Input: part model. Units: mm. Frame: model coordinates. A direction names the side the tool comes from. Give positions to 0.01 mm unless a question says otherwise; leave off trailing zeros. Order: outer loops, then holes, each group sorted by start corner. A loop starts at its lowest first (then second) coordinate and runs counter-clockwise, first axis right, second up. Notation, with made-up numbers: (-9.75, 55.25) - (3.25, 55.25) arc R23 cw to (3.25, 92.25) - close; hole circle Ø3 at (51.25, 19.25). An arc over 180 degrees is marked (long way). Answer in a Markdown table with one row per item. Add a question column.
1. Section query D-D on z = 7.5. Return loops of the section in (x, y).
2. Access query for faces 5 (the face through (0, -4, -10)), 6 (the face through (-0.13, -7.99, 8.49)), 7 (the face through (4.25, -4, 0)), 8 (the face through (-4.25, -4, 0)). Directions: +Z, -Z, +X, -X, +Y, -Y. A direction counts if a zero-diameter tool reaches every point of the face in a straight line with its end or side. Return the directions, or none.
3. Contact query for flat-ended pins moving along their axis: pin 1 (1.7 mm diameter, centred on y = -4, z = 2.5, fed in from +X); pin 2 (12 mm diameter, centred on x = 3.5, z = -5.5, fed in from -Y); pin 3 (12 mm diameter, centred on x = 4.5, z = -0.5, fed in from -Y); pin 4 (1 mm diameter, centred on x = -1.5, y = -6.5, fed in from -Z). Output: stop coordinate, or through.
4. Ray query, line 1 (Y direction, x = 9.5, z = 0); line 2 (Z direction, x = -1, y = -6); line 3 (X direction, y = -6, z = -8.25). Return the intervals inside material, ascending. Write a range as [from, to].
5. Section query B-B on x = 0. Return loops of the section in (y, z).
6. Mould query, pull axis Z, two halves, no side actions, for faces 1 (the face through (0, -4, 10)), 2 (the face through (6.586, -0.592, 10.329)), 3 (the face through (-0.13, -7.99, -6.51)), 4 (the face through (0, 0, 0)). Classes: released by +Z, released by -Z, zero draft, split by the parting line, or undercut.
7. Section query C-C on y = -3.25. Return loops of the section in (x, z).
8. Section query A-A on z = 0. Return loops of the section in (x, y).
```python
from build123d import *

# Parameters (mm, degrees)
F0_R     = 12.25
F0_W     = 8.5
F0_H     = 20
F1_DEPTH = 1.2
F0_R_2   = 1
F2_DEPTH = 7
F3_DEPTH = 9


with BuildPart() as f1:
    # F0 (on Front) → F1 (new body)
    with BuildSketch(Plane.XZ):
        Circle(F0_R)
        Rectangle(F0_W, F0_H, mode=Mode.SUBTRACT)
    extrude(amount=F1_DEPTH)

    # F0 (on Front) → F2 (join)
    with BuildSketch(Plane.XZ):
        Rectangle(F0_W, F0_H)
        with Locations((0, -7.5)):
            Circle(F0_R_2, mode=Mode.SUBTRACT)
        with Locations((0, 7.5)):
            Circle(F0_R_2, mode=Mode.SUBTRACT)
    extrude(amount=F2_DEPTH)

    # F0 (on Front) → F3 (join)
    with BuildSketch(Plane.XZ):
        with Locations((0, 7.5)):
            Circle(F0_R_2)
        with Locations((0, -7.5)):
            Circle(F0_R_2)
    extrude(amount=F3_DEPTH)


solid = f1.part
```
Answer:
| question | item | result |
|---|---|---|
| 1 | outline | (-9.69, -1.2) - (-4.25, -1.2) - (-4.25, -7) - (-1, -7) - (-1, -9) - (1, -9) - (1, -7) - (4.25, -7) - (4.25, -1.2) - (9.69, -1.2) - (9.69, 0) - (-9.69, 0) - close |
| 2 | face 5 | -Z, +X, -X, -Y |
| 2 | face 6 | -Y |
| 2 | face 7 | +Z, -Z, +X, -Y |
| 2 | face 8 | +Z, -Z, -X, -Y |
| 3 | pin 1 | stops at x = 4.25 |
| 3 | pin 2 | stops at y = -9 |
| 3 | pin 3 | stops at y = -7 |
| 3 | pin 4 | stops at z = -10 |
| 4 | line 1 | y = [-1.2, 0] |
| 4 | line 2 | z = [-10, 10] |
| 4 | line 3 | x = [-4.25, 4.25] |
| 5 | outline | (-9, -8.5) - (-7, -8.5) - (-7, -10) - (-1.2, -10) - (-1.2, -12.25) - (0, -12.25) - (0, 12.25) - (-1.2, 12.25) - (-1.2, 10) - (-7, 10) - (-7, 8.5) - (-9, 8.5) - (-9, 6.5) - (-7, 6.5) - (-7, -6.5) - (-9, -6.5) - close |
| 6 | face 1 | released by +Z |
| 6 | face 2 | split by the parting line |
| 6 | face 3 | undercut |
| 6 | face 4 | zero draft |
| 7 | outline | (-4.25, -10) - (4.25, -10) - (4.25, 10) - (-4.25, 10) - close |
| 8 | outline | (-12.25, -1.2) - (-4.25, -1.2) - (-4.25, -7) - (4.25, -7) - (4.25, -1.2) - (12.25, -1.2) - (12.25, 0) - (-12.25, 0) - close |
